```python
from build123d import *

# Parameters (mm, degrees)
F2_R = 12.85994464
F3_R = 1.1798499289
F4_R = 2.4039125508
F5_R = 0.4407061183
F6_R = 5


with BuildPart() as f1:
    # F0 (on Front) → F1 (revolve)
    with BuildSketch(Plane.XZ):
        Polygon((-10.0625008345, 0), (0, 0), (0, 17.7625007927), (-2.1874997765, 17.7625007927), (-6.3875010237, 14.0875000507), (-7.7875000425, 8.6625004187), (-6.3875010237, 7.0875007659), (-8.4875002503, 6.5625002608), align=None)
    revolve(axis=Axis((0, 0, 8.8812503964), (0, 0, -1)))

    # F2
    f2_edges = [f1.edges().sort_by_distance(p)[0] for p in [
        (6.387501, 0, 14.0875),
    ]]
    fillet(f2_edges, radius=F2_R)

    # F3
    f3_edges = [f1.edges().sort_by_distance(p)[0] for p in [
        (8.4875, 0, 6.5625),
    ]]
    fillet(f3_edges, radius=F3_R)

    # F4
    f4_edges = [f1.edges().sort_by_distance(p)[0] for p in [
        (7.7875, 0, 8.6625),
    ]]
    fillet(f4_edges, radius=F4_R)

    # F5
    f5_edges = [f1.edges().sort_by_distance(p)[0] for p in [
        (-6.661983, 0, 7.396293),
        (6.936463, 0, 7.705085),
        (6.387501, 0, 7.087501),
    ]]
    fillet(f5_edges, radius=F5_R)

    # F6
    f6_edges = [f1.edges().sort_by_distance(p)[0] for p in [
        (-2.792166, 0, 17.233418),
        (3.396831, 0, 16.704336),
        (2.1875, 0, 17.762501),
    ]]
    fillet(f6_edges, radius=F6_R)


solid = f1.part
```
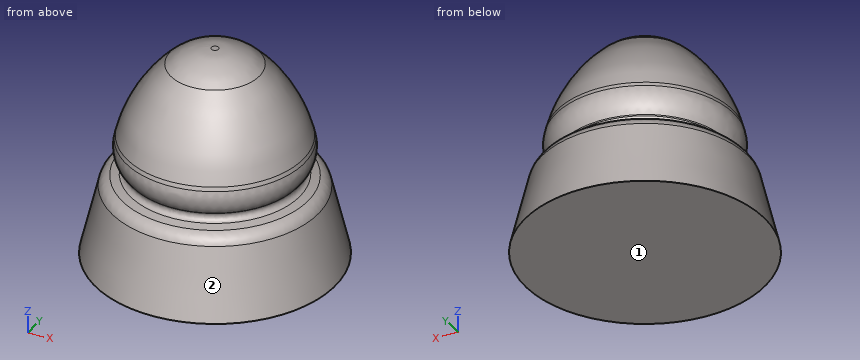
Verification items for the finished model (mm, model axes). Face numbers are marked on the shaded views. Coordinates: 2 decimals unless noted, no trailing zeros. Write each loop counter-clockwise with the first axis right and the second up, starting at its lowest first coordinate (ties: lowest second). Pieces come first, ordered by that corner, then holes. Notation, with made-up numbers: (-18.5, 43.5) - (20.5, 43.5) arc R24 ccw to (20.5, 54.5) - close; hole circle Ø11 at (-4, 45). An arc over 180 degrees is marked (long way). Write item = value, one per line.
Q1. Material ranges on L1, parallel to X at y = -2.25, z = 1.25; L2, parallel to X at y = 4.75, z = 9.5; L3, parallel to Y at x = 2.25, z = 5, recorded low to high. Write a range as from..to.
Answer:
L1 = -9.5..9.5
L2 = -5.85..5.85
L3 = -8.57..8.57
Q2. Mould release check, pull along Z, two halves, no side actions. Record for the marked faces 1 and 2: released by +Z, released by -Z, zero draft, split by the parting line, or undercut.
Answer:
face_1 = released by -Z
face_2 = released by +Z
Q3. Go/stop test with flat-tipped pins: pin 1 Ø3 at (y, z) = (-3, 3.5) entering from -X; pin 2 Ø5 at (x, z) = (-6.5, 3.5) entering from +Y; pin 3 Ø6 at (x, y) = (-7.5, 1) entering from +Z. Record where each tip stops, or that it passes through.
Answer:
pin_1 = -9.28
pin_2 = 8.48
pin_3 = 15.54
Q4. Cross-section at A-A (z = 5.25). Enter the section's corners in (x, y) (1 decimal), plus the area to 3 significant figures.
Answer:
outline = circle Ø17.6 at (0, 0)
area = 243 mm²
Q5. Cross-section at B-B (z = 1). Enter the section's corners in (x, y) (1 decimal), plus the area to 3 significant figures.
Answer:
outline = circle Ø19.6 at (0, 0)
area = 303 mm²
